from build123d import *

# Parameters (mm, degrees)
SKETCH1_R           = 2.5
BOSS_EXTRUDE1_DEPTH = 4
FILLET1_R           = 7.62


with BuildPart() as part:
    # Sketch1 → Boss-Extrude1 (new body)
    with BuildSketch(Plane(origin=(0, 25.4, 0), x_dir=(1, 0, 0), z_dir=(0, 1, 0))):
        Polygon((-127, -260.35), (-97.035940071, -260.35), (-76.2, -244.98413998), (-63.5, -244.98413998), (-63.5, -304.8), (-190.5, -304.8), (-190.5, -279.4), (-190.5, -260.35), (-165.1, -260.35), (-165.1, -279.4), (-127, -279.4), align=None)
        with Locations((-114.3, -292.1)):
            Circle(SKETCH1_R, mode=Mode.SUBTRACT)
        with Locations((-177.8, -292.1)):
            Circle(SKETCH1_R, mode=Mode.SUBTRACT)
        with Locations((-158.75, -292.1)):
            Circle(SKETCH1_R, mode=Mode.SUBTRACT)
        with Locations((-95.25, -292.1)):
            Circle(SKETCH1_R, mode=Mode.SUBTRACT)
        with Locations((-139.7, -292.1)):
            Circle(SKETCH1_R, mode=Mode.SUBTRACT)
        with Locations((-76.2, -292.1)):
            Circle(SKETCH1_R, mode=Mode.SUBTRACT)
        with Locations((-114.3, -273.05)):
            Circle(SKETCH1_R, mode=Mode.SUBTRACT)
        with Locations((-177.8, -273.05)):
            Circle(SKETCH1_R, mode=Mode.SUBTRACT)
        with Locations((-76.2, -260.35)):
            Circle(SKETCH1_R, mode=Mode.SUBTRACT)
    extrude(amount=BOSS_EXTRUDE1_DEPTH)

    # Fillet1
    fillet1_edges = [part.edges().sort_by_distance(p)[0] for p in [
        (-190.5, 27.4, 304.8),
        (-190.5, 27.4, 260.35),
        (-165.1, 27.4, 260.35),
        (-165.1, 27.4, 279.4),
        (-127, 27.4, 279.4),
        (-127, 27.4, 260.35),
        (-97.035940071, 27.4, 260.35),
        (-76.2, 27.4, 244.98413998),
        (-63.5, 27.4, 244.98413998),
        (-63.5, 27.4, 304.8),
    ]]
    fillet(fillet1_edges, radius=FILLET1_R)


solid = part.part
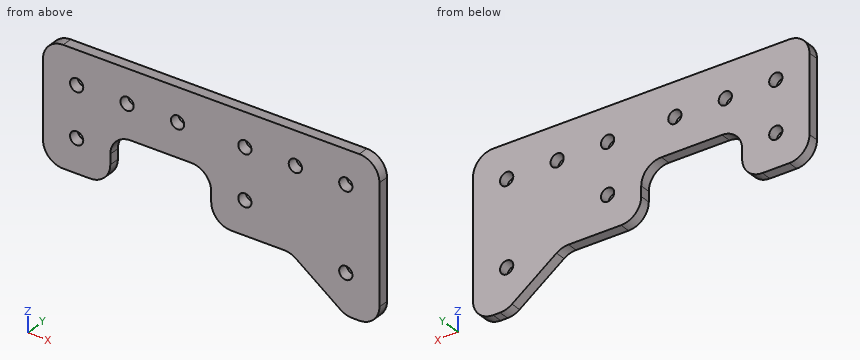
Build history of the part. All positions in model axes, mm. Coordinates: 2 decimals unless noted, no trailing zeros. Order: outer loops, then holes, each group sorted by start corner. A loop starts at its lowest first (then second) coordinate and runs counter-clockwise, first axis right, second up. Notation, with made-up numbers: M -3.5,-33.5 L 5.5,-33.5 A13 ccw 5.5,-8.5 Z; hole C -34.5,22 d6. An arc over 180 degrees is marked long. One line per question, with ' | ' between items. Start each with the question number.
Q1. Saw through at D-D (y = 26.55). Count the separate pieces of the cut face and the enclosed holes in it, then the cut area to 3 significant figures.
Q2. Saw through at C-C (x = -177.8). List the corners of the cut face in (y, z).
Q3. Saw through at B-B (z = 292.1). List the corners of the cut face in (x, y).
Q4. Saw through at A-A (x = -139.7). List the corners of the cut face in (y, z).
Q5. Flat gauge pins, fed straight in: pin 1 Ø1.5 at (x, y) = (-87.5, 27.5) entering from -Z; pin 2 Ø1.2 at (x, y) = (-177, 26.5) entering from -Z; pin 3 Ø1.2 at (x, y) = (-145, 27) entering from -Z. Where does each tip first touch, or does it go through?
Q6. Probe L1, parallel to Z at x = -177.8, y = 27.45; L2, parallel to X at y = 27.15, z = 273.05; L3, parallel to Z at x = -139.7, y = 26.4. List the from-to ranges inside material, lowest first. Write a range as from..to.
Check values:
1) separate pieces: 1 | enclosed holes: 9 | area: 5,050 mm2
2) outline: M 25.4,260.35 L 29.4,260.35 L 29.4,270.55 L 25.4,270.55 Z; M 25.4,275.55 L 29.4,275.55 L 29.4,289.6 L 25.4,289.6 Z; M 25.4,294.6 L 29.4,294.6 L 29.4,304.8 L 25.4,304.8 Z
3) outline: M -190.5,25.4 L -180.3,25.4 L -180.3,29.4 L -190.5,29.4 Z; M -175.3,25.4 L -161.25,25.4 L -161.25,29.4 L -175.3,29.4 Z; M -156.25,25.4 L -142.2,25.4 L -142.2,29.4 L -156.25,29.4 Z; M -137.2,25.4 L -116.8,25.4 L -116.8,29.4 L -137.2,29.4 Z; M -111.8,25.4 L -97.75,25.4 L -97.75,29.4 L -111.8,29.4 Z; M -92.75,25.4 L -78.7,25.4 L -78.7,29.4 L -92.75,29.4 Z; M -73.7,25.4 L -63.5,25.4 L -63.5,29.4 L -73.7,29.4 Z
4) outline: M 25.4,279.4 L 29.4,279.4 L 29.4,289.6 L 25.4,289.6 Z; M 25.4,294.6 L 29.4,294.6 L 29.4,304.8 L 25.4,304.8 Z
5) pin 1: stops at z = 252.76 | pin 2: stops at z = 260.35 | pin 3: stops at z = 279.4
6) L1: z = 260.35..270.55, 275.55..289.6, 294.6..304.8 | L2: x = -190.5..-180.3, -175.3..-164.99, -127.11..-116.8, -111.8..-63.5 | L3: z = 279.4..289.6, 294.6..304.8
